Input: part model. Units: mm. Frame: model coordinates. Face numbers are marked on the shaded views. A direction names the side the tool comes from. Round coordinates to 2 decimals unless told otherwise and drop trailing zeros. Loops run counter-clockwise (first coordinate to the right, second up) from the corner with the lowest first, then second, coordinate; pieces in that order, holes last. Notation, with made-up numbers: M 12,31 L 25,31 A16 ccw 25,42 Z; hole C 13,44 d11. An arc over 180 degrees is marked long. Put each result on its own line as item: value. Start each with the question number.
1) Reachability of the marked faces 1, 2, 3 and 4 from +Z, -Z, +X, -X, +Y, -Y: full face, straight path, thin tool, end or side. Return the list, or none.
2) Pin query (flat end, axial travel): pin 1 (9.5 mm diameter, centred on x = 1, z = 3.5, fed in from -Y); pin 2 (9 mm diameter, centred on x = -24, z = -19, fed in from -Y); pin 3 (2 mm diameter, centred on y = -4.5, z = 8.5, fed in from -X); pin 4 (3 mm diameter, centred on y = -4.5, z = -4, fed in from +X). Return the tip coordinate at first contact, or that it passes through.
3) Line query: probe 1 along Y at (x, z) = (-30, 16); probe 2 along X at (y, z) = (-6.5, -25.5); probe 3 along Y at (x, z) = (-5, 24.5). Output: solid intervals per line, ascending.
4) Section B-B on z = 0.5. Output: boundary loops of the cut face in (x, y).
5) Section C-C on x = 0. Output: boundary loops of the cut face in (y, z), plus the area to 3 significant figures.
6) Section A-A on y = -3.5. Output: boundary loops of the cut face in (x, z), plus the area to 3 significant figures.
from build123d import *

# Parameters (mm, degrees)
SKETCH1_W           = 78
SKETCH1_H           = 5
SKETCH1_W_2         = 4.5
BOSS_EXTRUDE2_DEPTH = 39
FILLET1_R           = 1


with BuildPart() as part:
    # Sketch1 → Boss-Extrude2 (new, symmetric)
    with BuildSketch(Plane.XY):
        Rectangle(SKETCH1_W, SKETCH1_H)
        with Locations((-6.65, -5)):
            Rectangle(SKETCH1_W_2, SKETCH1_H)
        with Locations((6.65, -5)):
            Rectangle(SKETCH1_W_2, SKETCH1_H)
    extrude(amount=BOSS_EXTRUDE2_DEPTH, both=True)

    # Fillet1
    fillet1_edges = [part.edges().sort_by_distance(p)[0] for p in [
        (0, 2.5, 39),
        (0, 2.5, -39),
        (8.9, -7.5, 0),
        (4.4, -7.5, 0),
        (-4.4, -7.5, 0),
        (-8.9, -7.5, 0),
        (-39, 2.5, 0),
        (39, 2.5, 0),
    ]]
    fillet(fillet1_edges, radius=FILLET1_R)


solid = part.part
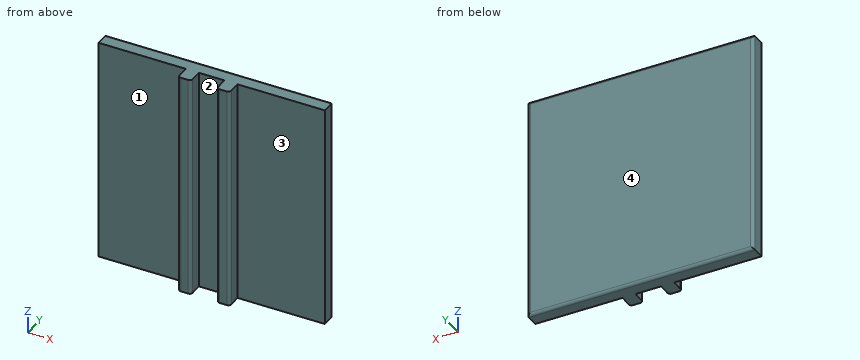
Geometry results:
1. face 1: +Z, -Z, -X, -Y
1. face 2: +Z, -Z, -Y
1. face 3: +Z, -Z, +X, -Y
1. face 4: +Z, -Z, +X, -X, +Y
2. pin 1: stops at y = -7.5
2. pin 2: stops at y = -2.5
2. pin 3: stops at x = -8.9
2. pin 4: stops at x = 8.9
3. probe 1: y = -2.5 to 2.5
3. probe 2: x = -8.9 to -4.4, 4.4 to 8.9
3. probe 3: y = -7.42 to 2.5
4. outline: M -39,-2.5 L -8.9,-2.5 L -8.9,-6.5 A1 ccw -7.9,-7.5 L -5.4,-7.5 A1 ccw -4.4,-6.5 L -4.4,-2.5 L 4.4,-2.5 L 4.4,-6.5 A1 ccw 5.4,-7.5 L 7.9,-7.5 A1 ccw 8.9,-6.5 L 8.9,-2.5 L 39,-2.5 L 39,1.5 A1 ccw 38,2.5 L -38,2.5 A1 ccw -39,1.5 Z
5. outline: M -2.5,-39 L 1.5,-39 A1 ccw 2.5,-38 L 2.5,38 A1 ccw 1.5,39 L -2.5,39 Z
5. area: 390 mm²
6. outline: M -8.9,-39 L -4.4,-39 L -4.4,39 L -8.9,39 Z; M 4.4,-39 L 8.9,-39 L 8.9,39 L 4.4,39 Z
6. area: 702 mm²
